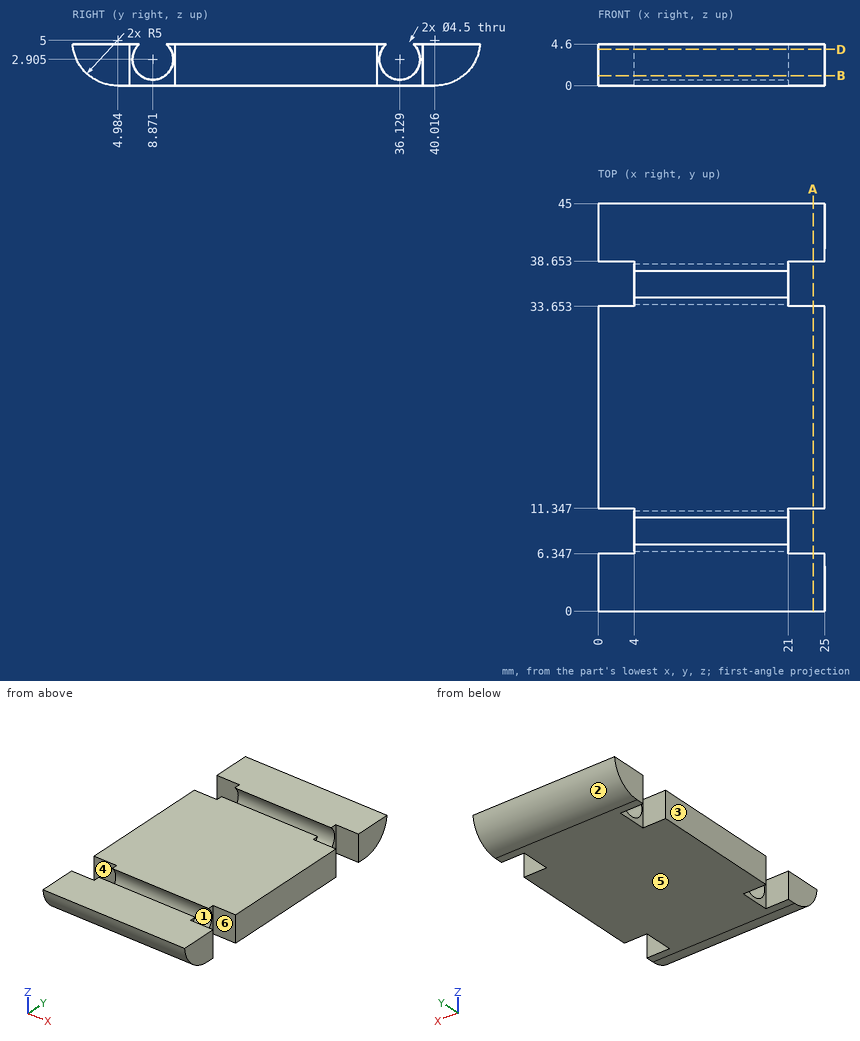
Drawing for the job (mm, zero at the part's lowest x, y, z). A direction names the side the tool comes from. Round coordinates to 2 decimals unless told otherwise and drop trailing zeros. Write each loop counter-clockwise with the first axis right and the second up, starting at its lowest first coordinate (ties: lowest second). Pieces come first, ordered by that corner, then holes. Notation, with made-up numbers: (25.5, 76) - (77.5, 76) arc R8 ccw to (77.5, 91) - close; hole circle Ø9 at (-3.5, -36.5). An arc over 180 degrees is marked (long way). Write item = value, one per line. Start each with the question number.
Q1. Band-saw the part on D-D (z = 4). Give the cut face in (x, y) (1 decimal), then the cut area to 3 significant figures.
Q2. Band-saw the part on B-B (z = 1.1). Give the cut face in (x, y) (1 decimal), then the cut area to 3 significant figures.
Q3. Which spindle directions (+Z, -Z, +X, -X, +Y, -Y) get a long thin tool onto all of the face, cutting with end or side? Do the marked faces 4, 5 and 6. Say none if no direction does.
Q4. Mould opens along Z. For the marked faces 1, 2 and 3 say: pulls with the +Z half, pulls with the -Z half, needs draft (parallel to the pull), parting line crosses it, or undercut.
Q5. Band-saw the part on A-A (x = 23.75). Give the cut face in (y, z).
Q6. Probe L1, parallel to Y at x = 17, z = 3.9 (1 decimal); L2, parallel to Y at x = 17.25, z = 1.7 (1 decimal); L3, parallel to X at y = 7, z = 1.1. List the from-to ranges inside material, lowest first. Write a range as from..to.
Q7. Drop flat-ended pins along their axis: pin 1 (2 mm diameter, centred on x = 22, z = 3, fed in from -Y) (1 decimal); pin 2 (1.2 mm diameter, centred on x = 1.5, z = 3.5, fed in from +Y) (1 decimal); pin 3 (2.5 mm diameter, centred on y = 36, z = 2, fed in from +X); pin 4 (2 mm diameter, centred on x = 22.5, z = 2, fed in from +Y). Give the stop position or say it passes through.
Answers below:
q1.outline = (0, 0.1) - (25, 0.1) - (25, 6.3) - (21, 6.3) - (21, 6.9) - (4, 6.9) - (4, 6.3) - (0, 6.3) - close; (0, 11.3) - (4, 11.3) - (4, 10.8) - (21, 10.8) - (21, 11.3) - (25, 11.3) - (25, 33.7) - (21, 33.7) - (21, 34.2) - (4, 34.2) - (4, 33.7) - (0, 33.7) - close; (0, 38.7) - (4, 38.7) - (4, 38.1) - (21, 38.1) - (21, 38.7) - (25, 38.7) - (25, 44.9) - (0, 44.9) - close
q1.area = 907 mm2
q2.outline = (0, 1.9) - (25, 1.9) - (25, 6.3) - (21, 6.3) - (21, 7.5) - (4, 7.5) - (4, 6.3) - (0, 6.3) - close; (0, 11.3) - (4, 11.3) - (4, 10.2) - (21, 10.2) - (21, 11.3) - (25, 11.3) - (25, 33.7) - (21, 33.7) - (21, 34.8) - (4, 34.8) - (4, 33.7) - (0, 33.7) - close; (0, 38.7) - (4, 38.7) - (4, 37.5) - (21, 37.5) - (21, 38.7) - (25, 38.7) - (25, 43.1) - (0, 43.1) - close
q2.area = 861 mm2
q3.face_4 = +Z, -Z, -X
q3.face_5 = -Z, +X, -X, +Y, -Y
q3.face_6 = +Z, -Z, +X
q4.face_1 = undercut
q4.face_2 = pulls with the -Z half
q4.face_3 = needs draft
q5.outline = (0, 4.6) arc R5 ccw to (4.98, 0) - (6.35, 0) - (6.35, 4.6) - close; (11.35, 0) - (33.65, 0) - (33.65, 4.6) - (11.35, 4.6) - close; (38.65, 0) - (40.02, 0) arc R5 ccw to (45, 4.6) - (38.65, 4.6) - close
q6.L1 = 0.1..6.9, 10.9..34.1, 38.1..44.9
q6.L2 = 1.2..7, 10.8..34.2, 38..43.8
q6.L3 = 4..21
q7.pin_1 = 0.1
q7.pin_2 = 44.9
q7.pin_3 = through
q7.pin_4 = 44.6
